Can you work these out from the drawing? Everything is in mm from the part's minimum corner. Coordinates: 2 decimals unless noted, no trailing zeros. Order: outer loops, then holes, each group sorted by start corner. A loop starts at its lowest first (then second) coordinate and runs counter-clockwise, first axis right, second up. Notation, with made-up numbers: (50, -38.5) -> (93, -38.5) arc R23 cw to (93, 0.5) -> close; hole circle Ø6 at (-21, -28). An arc over 180 degrees is marked (long way). Answer in a Markdown table with one row per item.
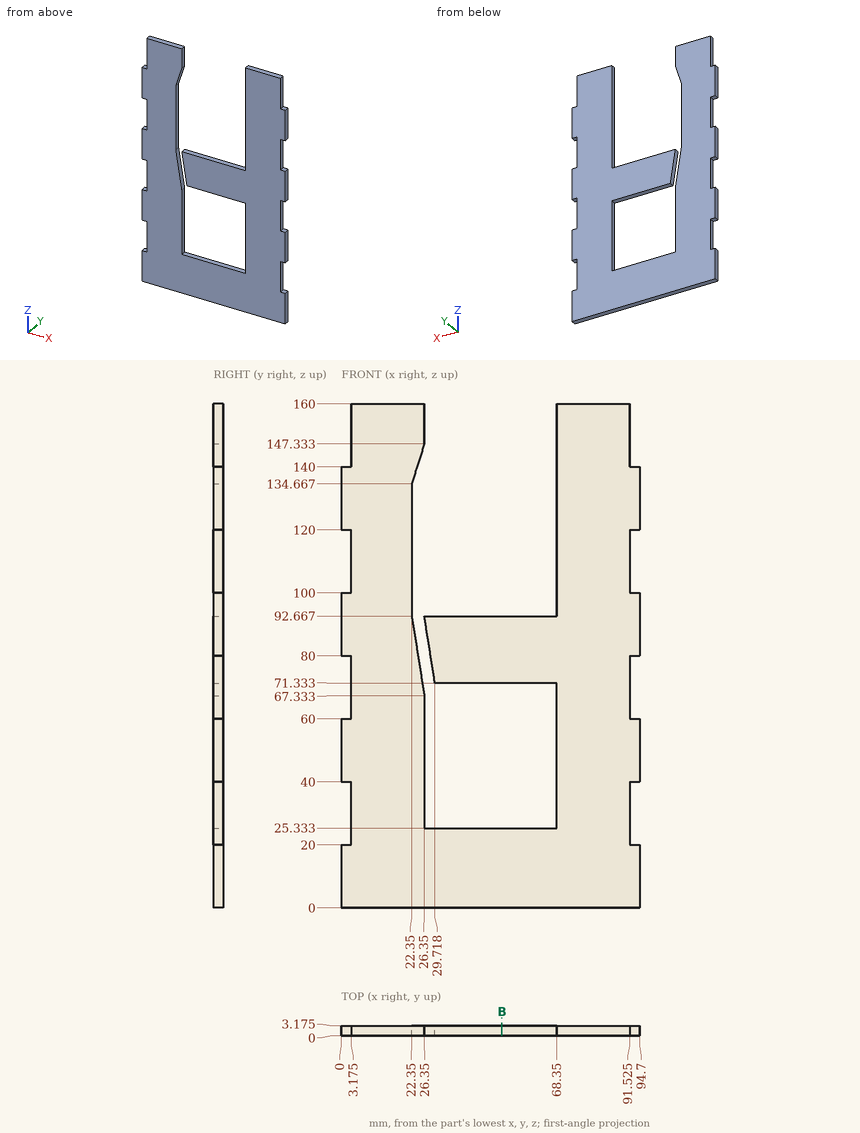
(1) I need wall thicknesses on line 1 (X direction, y = 2.1, z = 128); line 2 (X direction, y = 1.4, z = 55); line 3 (Z direction, x = 48, y = 2.85). Which ranges of each line are inside material? Lowest first, please. Write a range as [from, to].
Response values:
| item | result |
|---|---|
| line 1 | [0, 22.35], [68.35, 94.7] |
| line 2 | [0, 26.35], [68.35, 94.7] |
| line 3 | [0, 25.33], [71.33, 92.67] |
(2) Will these pins go through, and if not, where does the flat tip stop? pin 1 Ø1 at (y, z) = (1, 142) entering from -X (3 decimals); pin 2 Ø1 at (y, z) = (1.5, 154.5) entering from +X (3 decimals); pin 3 Ø1.5 at (x, y) = (55, 1) entering from +Z; pin 4 Ø4 at (x, z) = (25, 119) entering from +Y.
Response values:
| item | result |
|---|---|
| pin 1 | x = 3.175 |
| pin 2 | x = 91.525 |
| pin 3 | z = 92.67 |
| pin 4 | through |
(3) Suppose I cut it at B-B (x = 51). Please give me the cut outline in (y, z) (1 decimal), and give its area (3 significant figures).
Response values:
| item | result |
|---|---|
| outline | (0, 0) -> (3.2, 0) -> (3.2, 25.3) -> (0, 25.3) -> close; (0, 71.3) -> (3.2, 71.3) -> (3.2, 92.7) -> (0, 92.7) -> close |
| area | 148 mm2 |
